Part print with two shaded views. Sizes in mm from the minimum x, y, z corner. A direction names the side the tool comes from. Coordinates: 2 decimals unless noted, no trailing zeros. Order: outer loops, then holes, each group sorted by start corner. A loop starts at its lowest first (then second) coordinate and runs counter-clockwise, first axis right, second up.
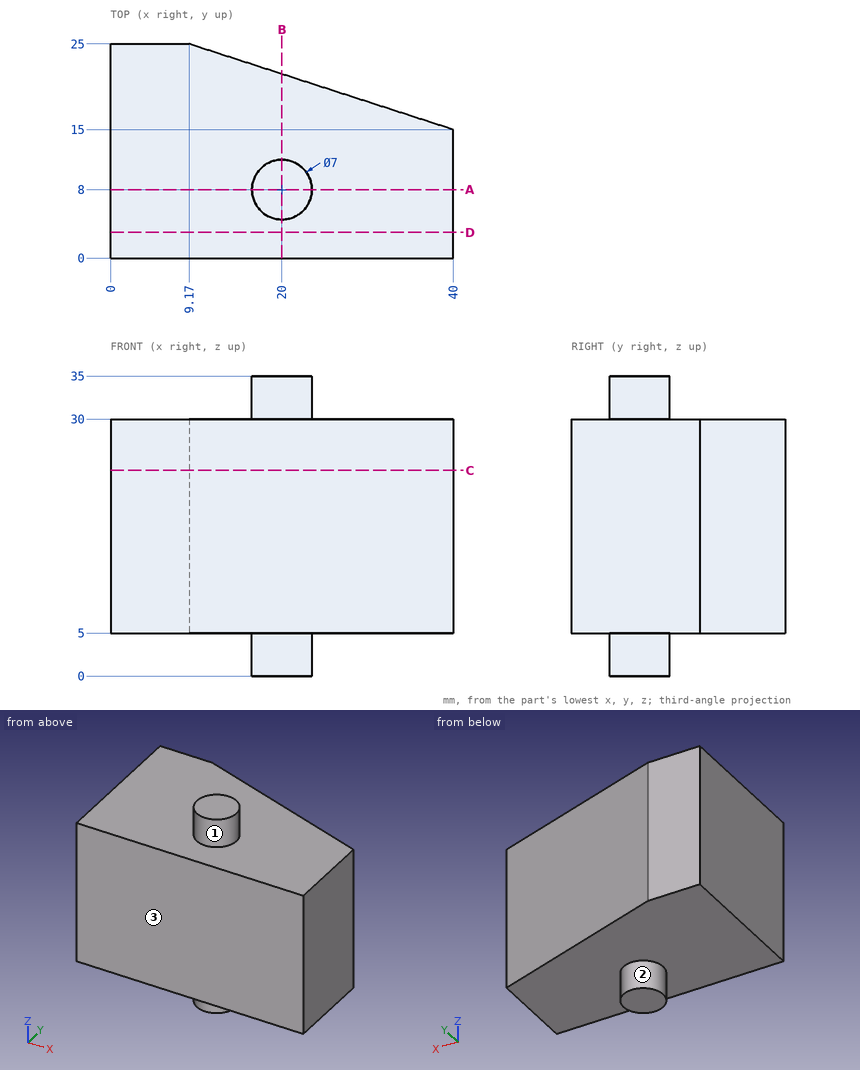
Q1. Wall check: line 1 along Z through (x, y) = (23.5, 18.5); line 2 along Y through (x, z) = (19.5, 16); line 3 along Y through (x, z) = (34, 29.5) (1 decimal). Give the ranges that are in metal, low to high.
Results list:
line 1: z = 5 to 30
line 2: y = 0 to 21.65
line 3: y = 0 to 16.9
Q2. Which spindle directions (+Z, -Z, +X, -X, +Y, -Y) get a long thin tool onto all of the face, cutting with end or side? Do the marked faces 1, 2 and 3. Say none if no direction does.
Results list:
face 1: +Z
face 2: -Z
face 3: +Z, -Z, +X, -X, -Y
Q3. Cut at B-B on x = 20. Write the cut outline in (y, z), and give its area (3 significant figures).
Results list:
outline: (0, 5) - (4.5, 5) - (4.5, 0) - (11.5, 0) - (11.5, 5) - (21.49, 5) - (21.49, 30) - (11.5, 30) - (11.5, 35) - (4.5, 35) - (4.5, 30) - (0, 30) - close
area: 607 mm2
Q4. Cut at A-A on y = 8. Write the cut outline in (x, z).
Results list:
outline: (0, 5) - (16.5, 5) - (16.5, 0) - (23.5, 0) - (23.5, 5) - (40, 5) - (40, 30) - (23.5, 30) - (23.5, 35) - (16.5, 35) - (16.5, 30) - (0, 30) - close
Q5. Pin check, flat tips, straight feed: pin 1 Ø4 at (x, z) = (20.5, 4) entering from +Y; pin 2 Ø10 at (x, y) = (21, 17) entering from +Z; pin 3 Ø7.5 at (x, y) = (28, 16.5) entering from -Z. Stop position of each tip, or through.
Results list:
pin 1: stops at y = 21.89
pin 2: stops at z = 30
pin 3: stops at z = 5
Q6. Cut at C-C on z = 24. Write the cut outline in (x, y).
Results list:
outline: (0, 0) - (40, 0) - (40, 15) - (9.17, 25) - (0, 25) - close
Q7. Cut at D-D on y = 3. Write the cut outline in (x, z), and give its area (3 significant figures).
Results list:
outline: (0, 5) - (40, 5) - (40, 30) - (0, 30) - close
area: 1,000 mm2
